Here's how the part is built. I have some questions about the finished solid (model axes, mm). A direction names the side the tool comes from. Coordinates: 2 decimals unless noted, no trailing zeros. Write each loop counter-clockwise with the first axis right and the second up, starting at its lowest first coordinate (ties: lowest second). Pieces come first, ordered by that corner, then holes. Notation, with made-up numbers: M 78,45 L 94,45 A23 ccw 94,71 Z; hole C -10,69.25 d4. An arc over 180 degrees is marked long. Use one line per item in the form item = value. Start each with the question number.
1. I want a section at A-A, the plane y = 5.75. Count the separate pieces of the cut face and the enclosed holes in it, plus the area to 3 significant figures.
2. I'm going to push flat-ended pins straight in: pin 1 Ø5 at (x, y) = (17, 14.5) entering from -Z; pin 2 Ø5 at (x, y) = (-29.5, 6.5) entering from +Z; pin 3 Ø6 at (x, y) = (31, 8) entering from +Z. Where does each tip first touch, or does it pass through?
3. Thinking about a two-plate mould opening in X: for faces 1 (the face through (44.943, 9.667, -9.98)), 2 (the face through (-53.067, 12.445, -0.086)), 3 (the face through (44.4, 17.78, -13.7)), 4 (the face through (-2.652, 13.71, -60.267)), which applies, released by +X, released by -X, zero draft, split by the parting line, or undercut?
4. I want a section at B-B, the plane z = 57. List the corners of the cut face in (x, y) for me (3 decimals).
5. On a 3-axis mill with a long thin cutter (end or side, diameter ignored), from which of +Z, -Z, +X, -X, +Y, -Y can I reach the whole of each face in a straight line? I mean faces 5 (the face through (-45.4, 0, -13.9)), 6 (the face through (59, 9.525, -15)), 7 (the face through (54.99, 5.73, 0.07)). Say none if no direction works.
6. Please list where these lines run through material, in increasing order: line 1 along X through (y, z) = (8.25, -53.34) (3 decimals); line 2 along Z through (x, y) = (-32.5, 8.5); line 3 along Z through (x, y) = (-20, 1.75). Write a range as [from, to].
7. I want a section at C-C, the plane x = 57. List the corners of the cut face in (y, z) for me (3 decimals).
from build123d import *

# Parameters (mm, degrees)
CHAMFER1_SIZE     = 1.778
CHAMFER1_SIZE2    = 1.111017708
CIRPATTERN1_COUNT = 4


with BuildPart() as part:
    # Sketch2 → Revolve1 (revolve)
    with BuildSketch(Plane.XY, mode=Mode.PRIVATE) as revolve1_sk:
        Polygon((-46.0375, 0), (-66.675, 0), (-66.675, 9.525), (-60.325, 9.525), (-60.325, 17.78), (-46.0375, 17.78), align=None)
    revolve(revolve1_sk.sketch.rotate(Axis((0, 0, 0), (0, -1, 0)), 270), axis=Axis((0, 0, 0), (0, -1, 0)))

    # Chamfer1
    chamfer1_edges = [part.edges().sort_by_distance(p)[0] for p in [
        (0, 0, -46.0375),
    ]]
    chamfer1_side = [part.faces().sort_by_distance(p)[0] for p in [
        (0, 8.89, -46.0375),
    ]]
    chamfer(chamfer1_edges, length=CHAMFER1_SIZE, length2=CHAMFER1_SIZE2, reference=chamfer1_side[0])

    # Sketch5 → M4x0.7 Tapped Hole2 (revolve, cut)
    with BuildSketch(Plane(origin=(0, 0, 53.34), x_dir=(0, 0, -1), z_dir=(1, 0, 0))):
        Polygon((0, 0), (0, 12.617000021), (1.65, 11.62558), (1.65, 0), align=None)
    m4x0_7_tapped_hole2 = revolve(axis=Axis((0, -6.35, 53.34), (0, 1, 0)), mode=Mode.SUBTRACT)

    # CirPattern1: M4x0.7 Tapped Hole2 ×4 about axis
    cirpattern1_axis = Axis((0, 0, 0), (0, 1, 0))
    for i in range(1, CIRPATTERN1_COUNT):
        add(m4x0_7_tapped_hole2.rotate(cirpattern1_axis, i * 360 / CIRPATTERN1_COUNT), mode=Mode.SUBTRACT)


solid = part.part
Answer list:
q1.separate_pieces = 1
q1.enclosed_holes = 5
q1.area = 7,270 mm²
q2.pin_1 = -58.56
q2.pin_2 = 60.96
q2.pin_3 = 60.51
q3.face_1 = undercut
q3.face_2 = undercut
q3.face_3 = zero draft
q3.face_4 = split by the parting line
q4.outline = M -34.591,0 L 34.591,0 L 34.591,9.525 L 19.751,9.525 L 19.751,17.78 L -19.751,17.78 L -19.751,9.525 L -34.591,9.525 Z
q5.face_5 = +Z, -Z, +X, -X, -Y
q5.face_6 = +Y
q5.face_7 = -Y
q6.line_1 = [-40.005, -1.65], [1.65, 40.005]
q6.line_2 = [-58.22, -32.61], [32.61, 58.22]
q6.line_3 = [-63.6, -41.49], [41.49, 63.6]
q7.outline = M 0,-34.591 L 9.525,-34.591 L 9.525,-19.751 L 17.78,-19.751 L 17.78,19.751 L 9.525,19.751 L 9.525,34.591 L 0,34.591 Z
